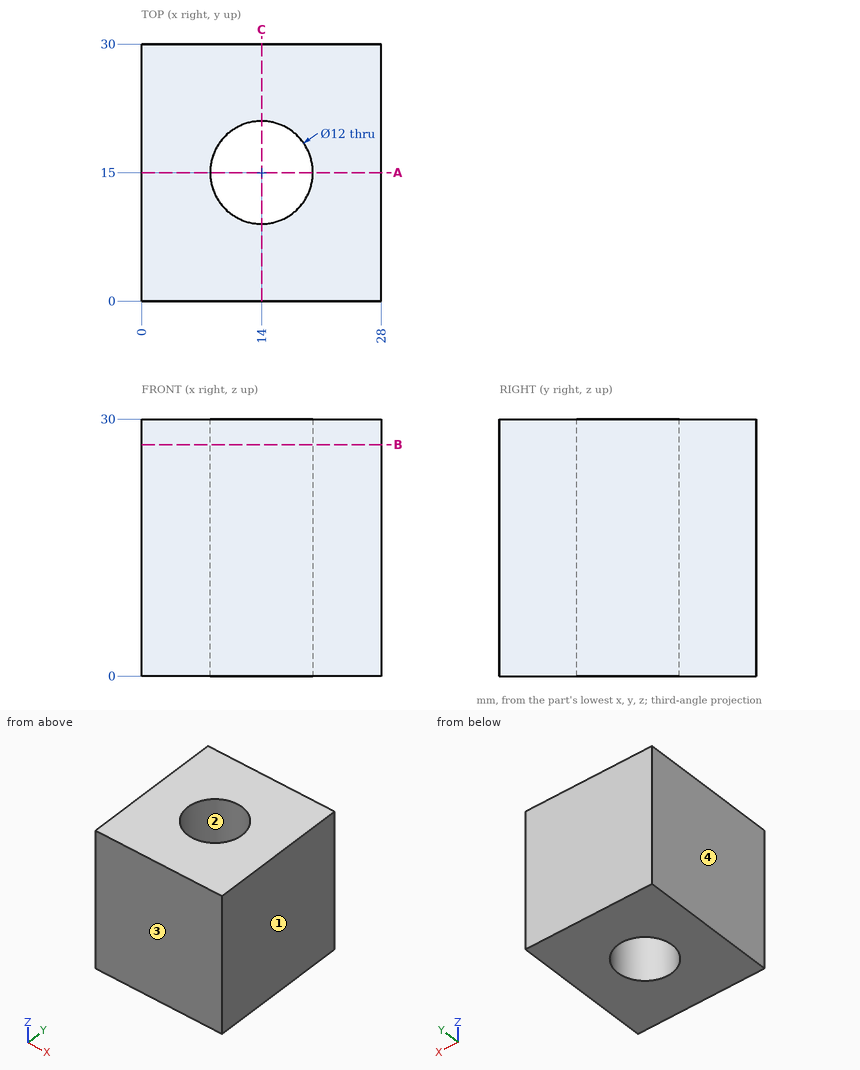
Geometry: see drawing. Coordinates: mm, zero at the bounding-box minimum. Coordinates: 2 decimals unless noted, no trailing zeros. Loops run counter-clockwise (first coordinate to the right, second up) from the corner with the lowest first, then second, coordinate; pieces in that order, holes last. Notation, with made-up numbers: (-38.5, 40.25) - (-17.5, 40.25) arc R22 ccw to (-17.5, 72.25) - close; hole circle Ø4 at (82.5, -29.5). An arc over 180 degrees is marked (long way). Return JSON: item names as keys, results as strings.
Q1. Section B-B, the plane z = 27. Return loops of the section in (x, y).
Results:
{"outline": "(0, 0) - (28, 0) - (28, 30) - (0, 30) - close; hole circle Ø12 at (14, 15)"}
Q2. Material intervals for line 1 along Y through (x, z) = (14, 22.25); line 2 along Y through (x, z) = (19.5, 25); line 3 along X through (y, z) = (13.5, 15.25), sorted ascending.
Results:
{"line 1": "0 to 9, 21 to 30", "line 2": "0 to 12.6, 17.4 to 30", "line 3": "0 to 8.19, 19.81 to 28"}
Q3. Section A-A, the plane y = 15. Return loops of the section in (x, z), plus the area to 3 significant figures.
Results:
{"outline": "(0, 0) - (8, 0) - (8, 30) - (0, 30) - close; (20, 0) - (28, 0) - (28, 30) - (20, 30) - close", "area": "480 mm2"}
Q4. Mould query, pull axis X, two halves, no side actions, for the marked faces 1, 2, 3 and 4. Classes: released by +X, released by -X, zero draft, split by the parting line, or undercut.
Results:
{"face 1": "released by +X", "face 2": "undercut", "face 3": "zero draft", "face 4": "released by -X"}
Q5. Contact query for flat-ended pins moving along their axis: P1, Ø1.5, axis at x = 3, y = 19.5, coming from the -Z side; P2, Ø7, axis at x = 14, y = 15, coming from the +Z side. Output: stop coordinate, or through.
Results:
{"P1": "z = 0", "P2": "through"}
Q6. Section C-C, the plane x = 14. Return loops of the section in (y, z).
Results:
{"outline": "(0, 0) - (9, 0) - (9, 30) - (0, 30) - close; (21, 0) - (30, 0) - (30, 30) - (21, 30) - close"}
